from build123d import *

# Parameters (mm, degrees)
SKETCH_1_R          = 4
EXTRUDE_1_DEPTH     = 30
SKETCH_6_R          = 2
CUT_EXTRUDE_5_DEPTH = 8
SKETCH_7_R          = 6
CUT_EXTRUDE_6_DEPTH = 2
CUT_EXTRUDE_START   = -2
SKETCH_8_R          = 6
CUT_EXTRUDE_7_DEPTH = 2


with BuildPart() as part:
    # 草图1 → 凸台-拉伸1 (new body)
    with BuildSketch(Plane(origin=(0, 0, 0), x_dir=(0, 0, -1), z_dir=(1, 0, 0))):
        with BuildLine():
            Line((-12.117188, -1), (-12.117188, -17))
            ThreePointArc((-12.117188, -17), (-11.824294782, -17.707106781), (-11.117188, -18))
            Line((-11.117188, -18), (20.882812, -18))
            ThreePointArc((20.882812, -18), (21.589918781, -17.707106781), (21.882812, -17))
            Line((21.882812, -17), (21.882812, -1))
            ThreePointArc((21.882812, -1), (21.589918781, -0.292893219), (20.882812, 0))
            Line((20.882812, 0), (13.297025562, 0))
            ThreePointArc((13.297025562, 0), (12.91434213, 0.076120467), (12.589918781, 0.292893219))
            Line((12.589918781, 0.292893219), (9.175705218, 3.707106781))
            ThreePointArc((9.175705218, 3.707106781), (8.85128187, 3.923879533), (8.468598437, 4))
            Line((8.468598437, 4), (1.297025562, 4))
            ThreePointArc((1.297025562, 4), (0.91434213, 3.923879533), (0.589918781, 3.707106781))
            Line((0.589918781, 3.707106781), (-2.824294782, 0.292893219))
            ThreePointArc((-2.824294782, 0.292893219), (-3.14871813, 0.076120467), (-3.531401563, 0))
            Line((-3.531401563, 0), (-11.117188, 0))
            ThreePointArc((-11.117188, 0), (-11.824294782, -0.292893219), (-12.117188, -1))
        make_face()
        with Locations((4.882812, -7)):
            Circle(SKETCH_1_R, mode=Mode.SUBTRACT)
    extrude(amount=EXTRUDE_1_DEPTH)

    # 草图6 → 切除-拉伸5 (cut)
    with BuildSketch(Plane.XZ.offset(18)):
        with Locations(Location((24, -16.882812, 0), (0, 0, 270))):
            Circle(SKETCH_6_R)
        with Locations(Location((6, -16.882812, 0), (0, 0, 270))):
            Circle(SKETCH_6_R)
        with Locations(Location((6, 7.117188, 0), (0, 0, 270))):
            Circle(SKETCH_6_R)
        with Locations(Location((24, 7.117188, 0), (0, 0, 270))):
            Circle(SKETCH_6_R)
    extrude(amount=-CUT_EXTRUDE_5_DEPTH, mode=Mode.SUBTRACT)

    # 草图7 → 切除-拉伸6 (cut)
    with BuildSketch(Plane.ZY):
        with Locations((-4.882812, -7)):
            Circle(SKETCH_7_R)
    extrude(amount=-CUT_EXTRUDE_6_DEPTH, mode=Mode.SUBTRACT)

    # 草图8 → 切除-拉伸7 (cut)
    with BuildSketch(Plane(origin=(30, 0, 0), x_dir=(0, 0, -1), z_dir=(1, 0, 0)).offset(CUT_EXTRUDE_START)):
        with Locations(Location((4.882812, -7, 0), (0, 0, 180))):
            Circle(SKETCH_8_R)
    extrude(amount=CUT_EXTRUDE_7_DEPTH, mode=Mode.SUBTRACT)


solid = part.part
Geometry check sheet. Reference: the model listing, model coordinates, mm. A direction names the side the tool comes from. Round coordinates to 2 decimals unless told otherwise and drop trailing zeros. Order: outer loops, then holes, each group sorted by start corner. A loop starts at its lowest first (then second) coordinate and runs counter-clockwise, first axis right, second up. Notation, with made-up numbers: M 21.5,48.25 L 60.5,48.25 A36 ccw 60.5,86.25 Z; hole C -27.5,64.25 d10. An arc over 180 degrees is marked long. Answer in a Markdown table with one row per item.
(1) Draft check along X on faces 4 (the face through (15, -9, -21.883)), 5 (the face through (30, -12, -1)), 6 (the face through (6, -10, 7)). Enter one of: released by +X, released by -X, zero draft, split by the parting line, or undercut.
Responses:
| item | result |
|---|---|
| face 4 | zero draft |
| face 5 | released by +X |
| face 6 | undercut |
(2) Go/stop test with flat-tipped pins: P1, Ø10.5, axis at y = -7, z = -4.88, coming from the -X side; P2, Ø3.5, axis at x = 6, z = 7.12, coming from the -Y side; P3, Ø9.5, axis at y = -8, z = -5, coming from the +X side; P4, Ø7, axis at y = -7, z = -4.88, coming from the +X side. Record where each tip stops, or that it passes through.
Responses:
| item | result |
|---|---|
| P1 | stops at x = 2 |
| P2 | stops at y = -10 |
| P3 | stops at x = 28 |
| P4 | passes through |
(3) Sectioned sample at B-B, the plane y = -7. Record the cut outline in (x, z), and give its area (3 significant figures).
Responses:
| item | result |
|---|---|
| outline | M 0,-21.88 L 30,-21.88 L 30,-10.88 L 28,-10.88 L 28,-8.88 L 2,-8.88 L 2,-10.88 L 0,-10.88 Z; M 0,1.12 L 2,1.12 L 2,-0.88 L 28,-0.88 L 28,1.12 L 30,1.12 L 30,12.12 L 0,12.12 Z |
| area | 764 mm² |
(4) Scan lines: probe 1 along Z at (x, y) = (7.75, -17); probe 2 along X at (y, z) = (-10.5, -18); probe 3 along Y at (x, z) = (16.5, 2). Record each from-to range of solid material in increasing order. Write a range as from..to.
Responses:
| item | result |
|---|---|
| probe 1 | z = -21.88..-17.85, -15.91..6.15, 8.09..12.12 |
| probe 2 | x = 0..4.34, 7.66..22.34, 25.66..30 |
| probe 3 | y = -18..1.12 |
(5) Sectioned sample at C-C, the plane y = -16.5. Record the cut outline in (x, z), and give its area (3 significant figures).
Responses:
| item | result |
|---|---|
| outline | M 0,-21.88 L 30,-21.88 L 30,12.12 L 0,12.12 Z; hole C 6,-16.88 d4; hole C 6,7.12 d4; hole C 24,-16.88 d4; hole C 24,7.12 d4 |
| area | 970 mm² |
(6) Sectioned sample at A-A, the plane x = 16.5. Record the cut outline in (y, z).
Responses:
| item | result |
|---|---|
| outline | M -18,-20.88 A1 ccw -17,-21.88 L -1,-21.88 A1 ccw 0,-20.88 L 0,-13.3 A1 cw 0.29,-12.59 L 3.71,-9.18 A1 ccw 4,-8.47 L 4,-1.3 A1 ccw 3.71,-0.59 L 0.29,2.82 A1 cw 0,3.53 L 0,11.12 A1 ccw -1,12.12 L -17,12.12 A1 ccw -18,11.12 Z; hole C -7,-4.88 d8 |
(7) Tool access check on faces 1 (the face through (24, -10, 7)), 2 (the face through (15, 0, 7)), 3 (the face through (0.986, -6.736, -10.877)). Record the directions out of +Z, -Z, +X, -X, +Y, -Y that give a thin tool (end or side, any length) a straight path to the whole face; none if there is none.
Responses:
| item | result |
|---|---|
| face 1 | -Y |
| face 2 | +Z, +X, -X, +Y |
| face 3 | -X |
(8) Sectioned sample at D-D, the plane z = -7. Record the cut outline in (x, y).
Responses:
| item | result |
|---|---|
| outline | M 0,-18 L 30,-18 L 30,-12.61 L 28,-12.61 L 28,-10.39 L 2,-10.39 L 2,-12.61 L 0,-12.61 Z; M 0,-1.39 L 2,-1.39 L 2,-3.61 L 28,-3.61 L 28,-1.39 L 30,-1.39 L 30,4 L 0,4 Z |
